Autodesk Fusion 360 part; units mm, degrees
sketch "Sketch1" plane through (0, 0, 0) normal (0, 0, 1) x (1, 0, 0)
  line L0 (-10, 72.4007) -> (12.5, 72.4007)
  line L1 (12.5, 72.4007) -> (12.5, -37.5993)
  line L2 (12.5, -37.5993) -> (-10, -37.5993)
  line L3 (-10, -37.5993) -> (-10, 72.4007)
  circle A0 centre (5, 64.9007) radius 2.5
  circle A1 centre (5, -30.0993) radius 2.5
  dimension "d1" = 5
  dimension "d2" = 5
  dimension "d3" = 95
  dimension "d4" = 15
  dimension "d5" = 7.5
  dimension "d6" = 7.5
  dimension "d7" = 7.5
extrude "Extrude1" add sketch "Sketch1" along normal blind 5
sketch "Sketch2" plane through (0, 0, 5) normal (0, 0, 1) x (-1, 0, 0)
  circle A0 centre (-5, -64.9007) radius 2.5
  circle A1 centre (-5, 30.0993) radius 2.5
  line L0 (10, 37.5993) -> (-12.5, 37.5993)
  line L1 (-12.5, 37.5993) -> (-12.5, -72.4007)
  line L2 (-12.5, -72.4007) -> (10, -72.4007)
  line L3 (10, -72.4007) -> (10, 37.5993)
  line L4 (10, -72.4007) -> (5, -72.4007)
  line L5 (5, -72.4007) -> (5, 37.5993)
  line L6 (5, 37.5993) -> (10, 37.5993)
  line L7 (10, 37.5993) -> (10, -72.4007)
  dimension "d10" = 5
extrude "Extrude2" add sketch "Sketch2" along normal blind 50.8 contours L0 L2 L3 L4 L5 L6 L7
sketch "Sketch3" plane through (-10, 0, 0) normal (-1, 0, 0) x (0, -1, 0)
  line L0 (-72.4007, 0) -> (37.5993, 0)
  line L1 (37.5993, 0) -> (37.5993, 55.8)
  line L2 (37.5993, 55.8) -> (-72.4007, 55.8)
  line L3 (-72.4007, 55.8) -> (-72.4007, 0)
  line L4 (-72.4007, 55.8) -> (37.5993, 55.8)
  line L5 (37.5993, 55.8) -> (37.5993, 50.8)
  line L6 (37.5993, 50.8) -> (-72.4007, 50.8)
  line L7 (-72.4007, 50.8) -> (-72.4007, 55.8)
  dimension "d13" = 5
extrude "Extrude3" add sketch "Sketch3" along normal blind 15 contours L1 L2 L3 L4 L5 L6 L7
sketch "Sketch4" plane through (0, 0, 50.8) normal (0, 0, -1) x (1, 0, 0)
  line L0 (-10, -72.4007) -> (-10, 37.5993)
  line L1 (-10, 37.5993) -> (-25, 37.5993)
  line L2 (-25, 37.5993) -> (-25, -72.4007)
  line L3 (-25, -72.4007) -> (-10, -72.4007)
  circle A0 centre (-17.5, 30.0993) radius 2.8953
  circle A1 centre (-17.5, -64.9007) radius 3.4334
  dimension "d16" = 95
  dimension "d17" = 7.5
  dimension "d18" = 7.5
extrude "Extrude4" cut sketch "Sketch4" against normal blind 20 contours A0 | A1
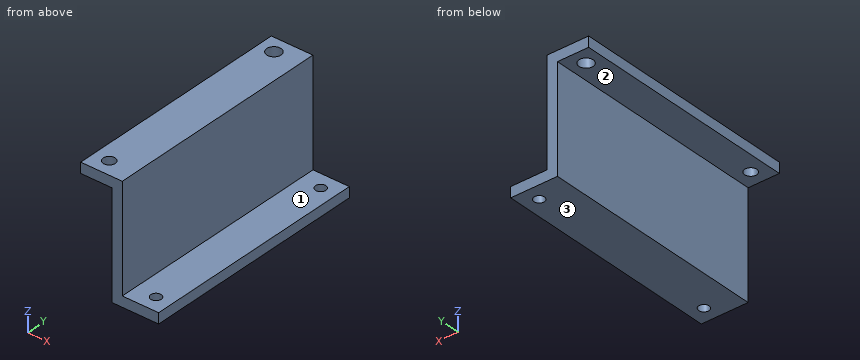
The listing builds one solid part. Answer for the finished solid, in the listing's coordinates (mm). Face numbers are marked on the shaded views. A direction names the side the tool comes from. Give positions to 0.01 mm unless a question says otherwise; leave off trailing zeros. Write each loop counter-clockwise with the first axis right and the second up, starting at its lowest first coordinate (ties: lowest second). Pieces come first, ordered by that corner, then holes.
1) Section A-A (x = 5) is taken. Write down the section's boundary in (y, z).
2) Section B-B (y = -10.5) is taken. Write down the section's boundary in (x, z), and give its area (4 significant figures).
3) Given P1, Ø1, axis at y = 36, z = 12.5, coming from the +X side; P2, Ø7.5, axis at x = -17.5, y = -30.1, coming from the -Z side; P3, Ø5, axis at x = 3.5, y = 21, coming from the +Z side, each flat-ended and moving along its own axis, determine where each tip first touches the part or whether it passes through.
4) A tool of negligible diameter and unlimited length cuts with its end or side. For the marked faces 1, 2 and 3, from which of +Z, -Z, +X, -X, +Y, -Y can it reach the whole face along a straight path? Write none if from no direction.
5) Find the intervals of material crossed by L1, parallel to Y at x = 5, z = 2.6; L2, parallel to Y at x = -18, z = 52.5; L3, parallel to Z at x = 0, y = 58.5, in increasing order.
6) Section C-C (x = -17.5) is taken. Write down the section's boundary in (y, z).
7) Section D-D (z = 38.5) is taken. Write down the section's boundary in (x, y).
Response:
1. outline: (-37.6, 0) - (-32.6, 0) - (-32.6, 5) - (-37.6, 5) - close; (-27.6, 0) - (62.4, 0) - (62.4, 5) - (-27.6, 5) - close; (67.4, 0) - (72.4, 0) - (72.4, 5) - (67.4, 5) - close
2. outline: (-25, 50.8) - (-10, 50.8) - (-10, 0) - (12.5, 0) - (12.5, 5) - (-5, 5) - (-5, 55.8) - (-25, 55.8) - close
2. area: 441.5 mm2
3. P1: stops at x = -5
3. P2: stops at z = 50.8
3. P3: stops at z = 5
4. face 1: +Z, +X, +Y, -Y
4. face 2: -Z, -X, +Y, -Y
4. face 3: -Z, +X, -X, +Y, -Y
5. L1: y = -37.6 to -32.6, -27.6 to 62.4, 67.4 to 72.4
5. L2: y = -37.6 to -32.95, -27.25 to 61.5, 68.3 to 72.4
5. L3: z = 0 to 5
6. outline: (-37.6, 50.8) - (-32.99, 50.8) - (-32.99, 55.8) - (-37.6, 55.8) - close; (-27.2, 50.8) - (61.47, 50.8) - (61.47, 55.8) - (-27.2, 55.8) - close; (68.33, 50.8) - (72.4, 50.8) - (72.4, 55.8) - (68.33, 55.8) - close
7. outline: (-10, -37.6) - (-5, -37.6) - (-5, 72.4) - (-10, 72.4) - close
